```python
from build123d import *

# Parameters (mm, degrees)
SKETCH1_W           = 280
SKETCH1_H           = 120
BOSS_EXTRUDE1_DEPTH = 5
SKETCH1_3_W         = 10
SKETCH1_3_H         = 40
CUT_EXTRUDE1_DEPTH  = 134
SKETCH1_4_W         = 10
SKETCH1_4_H         = 40
CUT_EXTRUDE2_DEPTH  = 229
SKETCH4_W           = 70
SKETCH4_H           = 8
CUT_EXTRUDE4_DEPTH  = 229
SKETCH3_W           = 4
SKETCH3_H           = 12
SKETCH3_W_2         = 12
SKETCH3_H_2         = 3
CUT_EXTRUDE5_DEPTH  = 10


with BuildPart() as part:
    # Sketch1 → Boss-Extrude1 (new body)
    with BuildSketch(Plane(origin=(0, 0, 0), x_dir=(1, 0, 0), z_dir=(0, 1, 0))):
        with Locations((140, 60)):
            Rectangle(SKETCH1_W, SKETCH1_H)
    extrude(amount=BOSS_EXTRUDE1_DEPTH)

    # Sketch1<3> → Cut-Extrude1 (cut)
    with BuildSketch(Plane(origin=(0, 0, 0), x_dir=(1, 0, 0), z_dir=(0, 1, 0))):
        with Locations((227, 95.54438009)):
            Rectangle(SKETCH1_3_W, SKETCH1_3_H)
        with Locations((227, 25.54438009)):
            Rectangle(SKETCH1_3_W, SKETCH1_3_H)
        with Locations((197, 25.54438009)):
            Rectangle(SKETCH1_3_W, SKETCH1_3_H)
        with Locations((167, 25.54438009)):
            Rectangle(SKETCH1_3_W, SKETCH1_3_H)
        with Locations((167, 95.54438009)):
            Rectangle(SKETCH1_3_W, SKETCH1_3_H)
        with Locations((137, 95.54438009)):
            Rectangle(SKETCH1_3_W, SKETCH1_3_H)
        with Locations((107, 95.54438009)):
            Rectangle(SKETCH1_3_W, SKETCH1_3_H)
        with Locations((107, 25.54438009)):
            Rectangle(SKETCH1_3_W, SKETCH1_3_H)
        with Locations((77, 25.54438009)):
            Rectangle(SKETCH1_3_W, SKETCH1_3_H)
        with Locations((47, 95.54438009)):
            Rectangle(SKETCH1_3_W, SKETCH1_3_H)
        with Locations((47, 25.54438009)):
            Rectangle(SKETCH1_3_W, SKETCH1_3_H)
        with Locations((257, 95.54438009)):
            Rectangle(SKETCH1_3_W, SKETCH1_3_H)
        with Locations((257, 25.54438009)):
            Rectangle(SKETCH1_3_W, SKETCH1_3_H)
        with Locations((197, 95.54438009)):
            Rectangle(SKETCH1_3_W, SKETCH1_3_H)
        with Locations((137, 25.54438009)):
            Rectangle(SKETCH1_3_W, SKETCH1_3_H)
        with Locations((77, 95.54438009)):
            Rectangle(SKETCH1_3_W, SKETCH1_3_H)
        with Locations((17, 25.54438009)):
            Rectangle(SKETCH1_3_W, SKETCH1_3_H)
    extrude(amount=CUT_EXTRUDE1_DEPTH, mode=Mode.SUBTRACT)

    # Sketch1<4> → Cut-Extrude2 (cut)
    with BuildSketch(Plane(origin=(0, 0, 0), x_dir=(1, 0, 0), z_dir=(0, 1, 0))):
        with Locations((17, 95.54438009)):
            Rectangle(SKETCH1_4_W, SKETCH1_4_H)
    extrude(amount=CUT_EXTRUDE2_DEPTH, mode=Mode.SUBTRACT)

    # Sketch4 → Cut-Extrude4 (cut)
    with BuildSketch(Plane(origin=(0, 5, 0), x_dir=(1, 0, 0), z_dir=(0, 1, 0))):
        with Locations((136.177664652, 61.117706899)):
            Rectangle(SKETCH4_W, SKETCH4_H)
        with Locations((46.177664652, 61.117706899)):
            Rectangle(SKETCH4_W, SKETCH4_H)
        with Locations((226.177664652, 61.117706899)):
            Rectangle(SKETCH4_W, SKETCH4_H)
    extrude(amount=-CUT_EXTRUDE4_DEPTH, mode=Mode.SUBTRACT)

    # Sketch3 → Cut-Extrude5 (cut)
    with BuildSketch(Plane(origin=(0, 5, 0), x_dir=(1, 0, 0), z_dir=(0, 1, 0))):
        with Locations((278, 11.128497482)):
            Rectangle(SKETCH3_W, SKETCH3_H)
        with Locations((30.63115044, 1.5)):
            Rectangle(SKETCH3_W_2, SKETCH3_H_2)
        with Locations((74.910678106, 1.5)):
            Rectangle(SKETCH3_W_2, SKETCH3_H_2)
        with Locations((122.372965913, 1.5)):
            Rectangle(SKETCH3_W_2, SKETCH3_H_2)
        with Locations((157.627034087, 1.5)):
            Rectangle(SKETCH3_W_2, SKETCH3_H_2)
        with Locations((209.75390842, 1.5)):
            Rectangle(SKETCH3_W_2, SKETCH3_H_2)
        with Locations((249.36884956, 1.5)):
            Rectangle(SKETCH3_W_2, SKETCH3_H_2)
        with Locations((278, 45.895590182)):
            Rectangle(SKETCH3_W, SKETCH3_H)
        with Locations((278, 105.740728373)):
            Rectangle(SKETCH3_W, SKETCH3_H)
        with Locations((278, 76.34695717)):
            Rectangle(SKETCH3_W, SKETCH3_H)
        with Locations((249.36884956, 118.5)):
            Rectangle(SKETCH3_W_2, SKETCH3_H_2)
        with Locations((209.75390842, 118.5)):
            Rectangle(SKETCH3_W_2, SKETCH3_H_2)
        with Locations((157.627034087, 118.5)):
            Rectangle(SKETCH3_W_2, SKETCH3_H_2)
        with Locations((122.372965913, 118.5)):
            Rectangle(SKETCH3_W_2, SKETCH3_H_2)
        with Locations((74.910678106, 118.5)):
            Rectangle(SKETCH3_W_2, SKETCH3_H_2)
        with Locations((30.63115044, 118.5)):
            Rectangle(SKETCH3_W_2, SKETCH3_H_2)
        with Locations((2, 105.740728373)):
            Rectangle(SKETCH3_W, SKETCH3_H)
        with Locations((2, 76.34695717)):
            Rectangle(SKETCH3_W, SKETCH3_H)
        with Locations((2, 45.895590182)):
            Rectangle(SKETCH3_W, SKETCH3_H)
        with Locations((2, 11.128497482)):
            Rectangle(SKETCH3_W, SKETCH3_H)
    extrude(amount=-CUT_EXTRUDE5_DEPTH, mode=Mode.SUBTRACT)


solid = part.part
```
Geometry check sheet. Reference: the model listing, model coordinates, mm. A direction names the side the tool comes from. Coordinates: 2 decimals unless noted, no trailing zeros. Write each loop counter-clockwise with the first axis right and the second up, starting at its lowest first coordinate (ties: lowest second). Pieces come first, ordered by that corner, then holes. Notation, with made-up numbers: (3.25, -17) -> (40.25, -17) arc R23 cw to (40.25, 14) -> close; hole circle Ø11 at (-28.5, 8). An arc over 180 degrees is marked (long way). Use CSV: the item, a comma, the result in double quotes. Start each with the question number.
Item 1: Depth check by flat-ended pin: pin 1 Ø1.5 at (x, y) = (120, 3) entering from -Z; pin 2 Ø2.5 at (y, z) = (1.5, -107) entering from +X; pin 3 Ø1 at (x, y) = (246.5, 1) entering from +Z. Enter the tip coordinate at first touch or a pass-through.
Item 2: Cross-section at B-B, the plane z = -33.5. State how many separate pieces and enclosed holes the cut face has, plus the area to 3 significant figures.
Item 3: Thickness scan on line 1 (Z direction, x = 73, y = 1.75); line 2 (Z direction, x = 168, y = 0.25); line 3 (Z direction, x = 250, y = 3). Record the ranges inside material, lowest first.
Item 4: Mould release check, pull along Z, two halves, no side actions. Record for faces 1 (the flat face through (158, 3, -117)), 2 (the flat face through (280, 2, -28)), 3 (the flat face through (232, 2, -25)), 4 (the flat face through (257, 2, -5.544)): released by +Z, released by -Z, zero draft, split by the parting line, or undercut.
Item 5: Set-up check for faces 5 (the flat face through (137, 2, -5.544)), 6 (the flat face through (4, 3, -11)), 7 (the flat face through (98, 2, -120)), 8 (the flat face through (276, 3, -106)): record each of +Z, -Z, +X, -X, +Y, -Y from which the full face is reachable in a straight line by a thin tool's end or side.
Item 6: Cross-section at A-A, the plane x = 239. Record the cut outline in (y, z).
Answers:
1,pin 1,"z = -117"
1,pin 2,"x = 276"
1,pin 3,"z = -3"
2,separate pieces,"10"
2,enclosed holes,"0"
2,area,"950 mm^2"
3,line 1,"-117 to -115.54, -75.54 to -65.12, -57.12 to -45.54, -5.54 to -3"
3,line 2,"-120 to -115.54, -75.54 to -65.12, -57.12 to -45.54, -5.54 to 0"
3,line 3,"-117 to -65.12, -57.12 to -3"
4,face 1,"released by -Z"
4,face 2,"zero draft"
4,face 3,"undercut"
4,face 4,"undercut"
5,face 5,"+Y, -Y"
5,face 6,"-X, +Y, -Y"
5,face 7,"-Z, +X, -X, +Y, -Y"
5,face 8,"+X, +Y, -Y"
6,outline,"(0, -120) -> (5, -120) -> (5, -65.12) -> (0, -65.12) -> close; (0, -57.12) -> (5, -57.12) -> (5, 0) -> (0, 0) -> close"
